Verification items for this drawing (mm, ordinates from the low corner). A direction names the side the tool comes from. Coordinates: 2 decimals unless noted, no trailing zeros. Loops run counter-clockwise (first coordinate to the right, second up) from the corner with the lowest first, then second, coordinate; pieces in that order, holes last. Notation, with made-up numbers: (1, -18.75) -> (6, -18.75) arc R4 cw to (6, -14.75) -> close; hole circle Ø3 at (54.25, 36.5). An arc over 180 degrees is marked (long way). Write item = value, one per line.
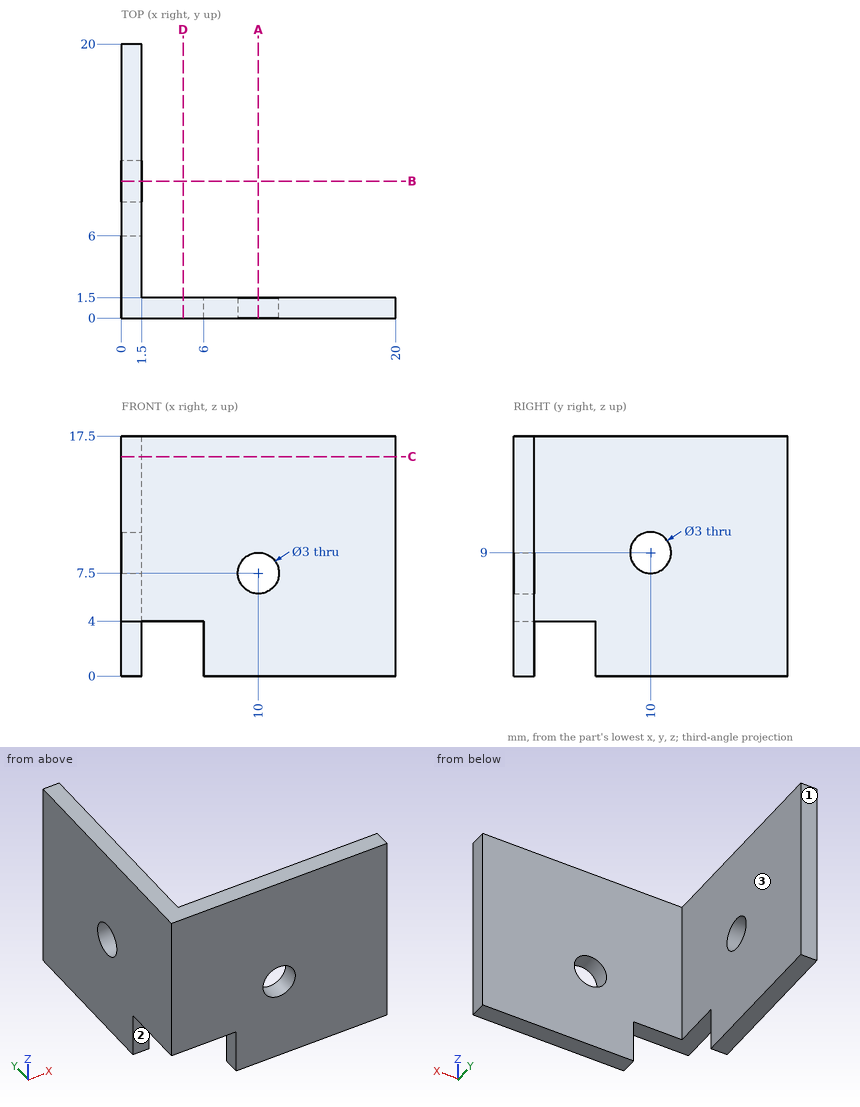
1) Sectioned sample at C-C, the plane z = 16. Record the cut outline in (x, y), plus the area to 4 significant figures.
Ans:
outline = (0, 0) -> (20, 0) -> (20, 1.5) -> (1.5, 1.5) -> (1.5, 20) -> (0, 20) -> close
area = 57.75 mm2
2) Tool access check on the marked faces 1, 2 and 3. Record the directions out of +Z, -Z, +X, -X, +Y, -Y that give a thin tool (end or side, any length) a straight path to the whole face; none if there is none.
Ans:
face_1 = +Z, -Z, +X, -X, +Y
face_2 = -Z, +X, -X, -Y
face_3 = +Z, -Z, +X, +Y
3) Sectioned sample at B-B, the plane y = 10. Record the cut outline in (x, z).
Ans:
outline = (0, 0) -> (1.5, 0) -> (1.5, 7.5) -> (0, 7.5) -> close; (0, 10.5) -> (1.5, 10.5) -> (1.5, 17.5) -> (0, 17.5) -> close
4) Sectioned sample at D-D, the plane x = 4.5. Record the cut outline in (y, z), plus the area to 4 significant figures.
Ans:
outline = (0, 4) -> (1.5, 4) -> (1.5, 17.5) -> (0, 17.5) -> close
area = 20.25 mm2
5) Depth check by flat-ended pin: pin 1 Ø1 at (y, z) = (15.5, 8) entering from +X; pin 2 Ø9 at (x, z) = (12.5, 7.5) entering from +Y; pin 3 Ø0.8 at (y, z) = (0.5, 2) entering from -X. Enter the tip coordinate at first touch or a pass-through.
Ans:
pin_1 = 1.5
pin_2 = 1.5
pin_3 = 6
6) Material ranges on line 1 (Z direction, x = 1.15, y = 10); line 2 (Z direction, x = 10, y = 0.9); line 3 (Y direction, x = 16.5, z = 14), recorded low to high.
Ans:
line_1 = 0 to 7.5, 10.5 to 17.5
line_2 = 0 to 6, 9 to 17.5
line_3 = 0 to 1.5
7) Sectioned sample at A-A, the plane x = 10. Record the cut outline in (y, z).
Ans:
outline = (0, 0) -> (1.5, 0) -> (1.5, 6) -> (0, 6) -> close; (0, 9) -> (1.5, 9) -> (1.5, 17.5) -> (0, 17.5) -> close
